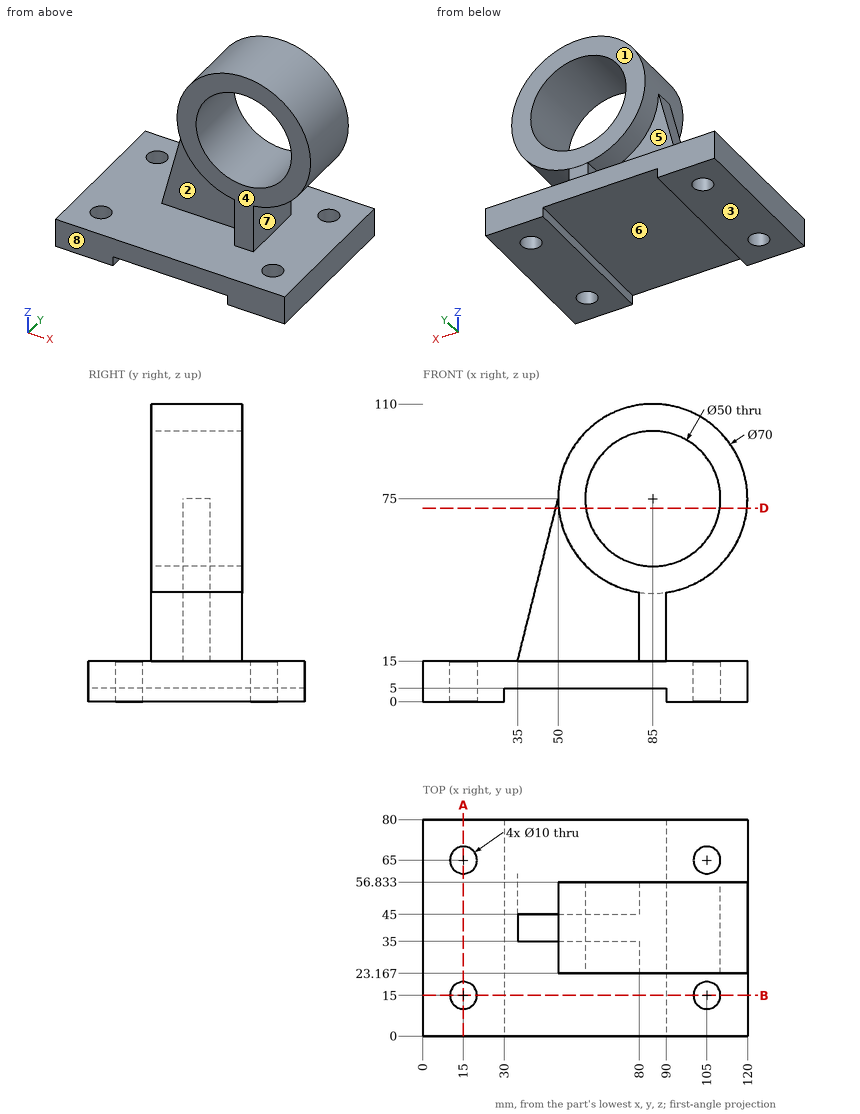
For this review, use the dimensioned drawing (mm, ordinates from the lowest corner) and the shaded views. A direction names the side the tool comes from. Round coordinates to 2 decimals unless told otherwise and drop trailing zeros. Order: outer loops, then holes, each group sorted by start corner. A loop starts at its lowest first (then second) coordinate and runs counter-clockwise, first axis right, second up. Notation, with made-up numbers: M 82,12.25 L 116,12.25 A14 ccw 116,18.25 Z; hole C 5.5,-34.75 d5. An arc over 180 degrees is marked long. Use a Markdown table: item, result.
1) Wall thickness on line 1 along Y through (x, z) = (15, 9); line 2 along Z through (x, y) = (85, 43); line 3 along Z through (x, y) = (41.5, 33): over which ranges is each line inside the solid? List them lowest first. Write a range as [from, to].
Report:
| item | result |
|---|---|
| line 1 | [0, 10], [20, 60], [70, 80] |
| line 2 | [5, 50], [100, 110] |
| line 3 | [5, 15] |
2) Insertion check: pin 1 (13.5 mm diameter, centred on x = 54.5, z = 43.5, fed in from +Y); pin 2 (8 mm diameter, centred on y = 26.5, z = 30.5, fed in from -X); pin 3 (10 mm diameter, centred on x = 52.5, y = 15.5, fed in from +Z). Each pin has a flat end and moves straight along its axis. Give the tip position at first contact, or say it passes through.
Report:
| item | result |
|---|---|
| pin 1 | y = 45 |
| pin 2 | x = 80 |
| pin 3 | z = 15 |
3) Consider section B-B (y = 15). Write out the cut boundary in (x, z).
Report:
| item | result |
|---|---|
| outline | M 0,0 L 10,0 L 10,15 L 0,15 Z; M 20,0 L 30,0 L 30,5 L 90,5 L 90,0 L 100,0 L 100,15 L 20,15 Z; M 110,0 L 120,0 L 120,15 L 110,15 Z |
4) Draft analysis for pull direction X (two halves, no side actions). For the marked faces 6, 7 and 8, state which applies: released by +X, released by -X, zero draft, split by the parting line, or undercut.
Report:
| item | result |
|---|---|
| face 6 | undercut |
| face 7 | released by +X |
| face 8 | zero draft |
5) Consider section D-D (z = 71.5). Write out the cut boundary in (x, y) (1 decimal).
Report:
| item | result |
|---|---|
| outline | M 49.1,35 L 50.2,35 L 50.2,23.2 L 60.2,23.2 L 60.2,56.8 L 50.2,56.8 L 50.2,45 L 49.1,45 Z; M 109.8,23.2 L 119.8,23.2 L 119.8,56.8 L 109.8,56.8 Z |
6) Tool access review of the marked faces 1, 2, 3, 4 and 5: name each direction out of +Z, -Z, +X, -X, +Y, -Y from which nothing blocks a thin tool from reaching the whole face with its end or side.
Report:
| item | result |
|---|---|
| face 1 | +Z, +X, -X, +Y |
| face 2 | -X, -Y |
| face 3 | -Z, +X, -X, +Y, -Y |
| face 4 | +Z, +X, -X, -Y |
| face 5 | -X, +Y |
7) Consider section A-A (x = 15). Write out the cut boundary in (y, z).
Report:
| item | result |
|---|---|
| outline | M 0,0 L 10,0 L 10,15 L 0,15 Z; M 20,0 L 60,0 L 60,15 L 20,15 Z; M 70,0 L 80,0 L 80,15 L 70,15 Z |
